Could you check a few things on this drawing? It's one solid part, dimensions in mm from its lowest x, y, z. A direction names the side the tool comes from. Give positions to 0.01 mm unless a question says otherwise; leave off trailing zeros. Loops run counter-clockwise (first coordinate to the right, second up) from the corner with the lowest first, then second, coordinate; pieces in that order, holes last. Notation, with made-up numbers: (-23, 11.5) - (34, 11.5) arc R29 cw to (34, 31.5) - close; hole circle Ø1 at (59.5, 68). An arc over 180 degrees is marked (long way). Use CSV: the item, a comma, the result in double quotes.
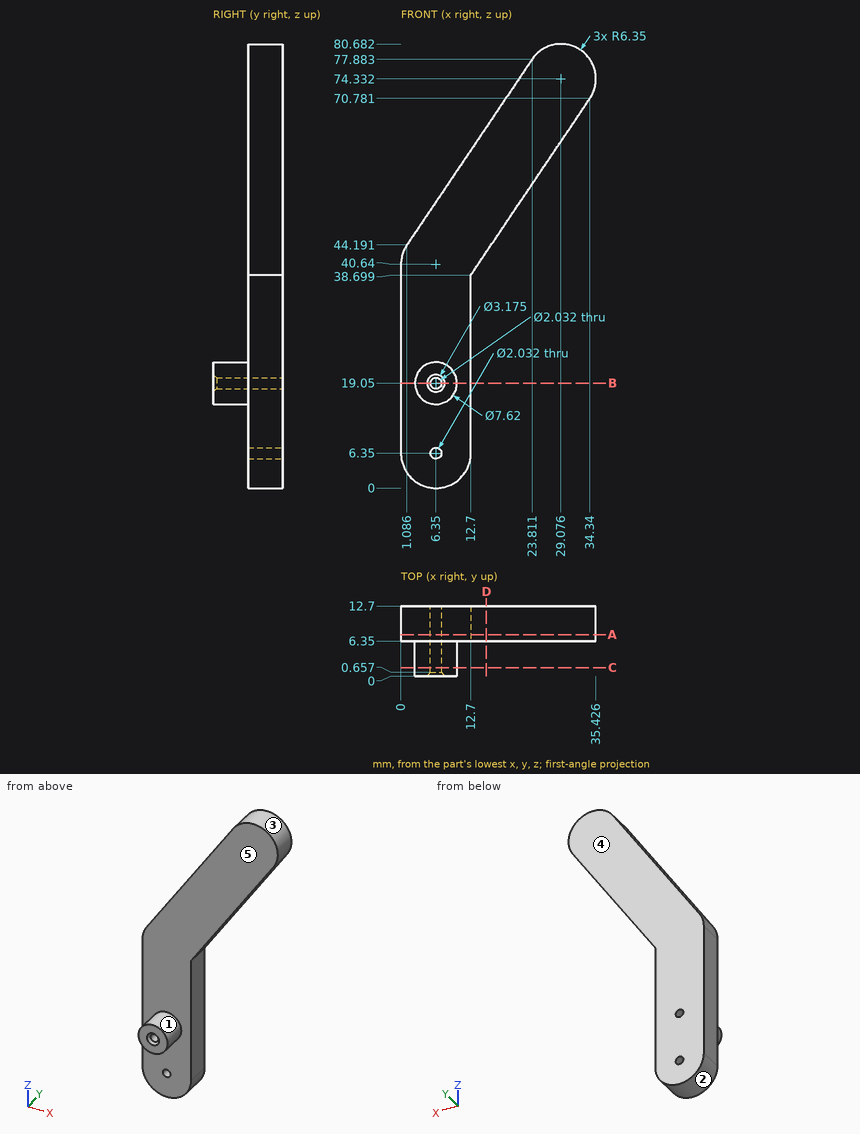
1) Which directions (+Z, -Z, +X, -X, +Y, -Y) give clear straight access to the entire face, cutting with the end or side of a thin tool? Please do the marked faces 1 and 2.
Answer below:
face 1,"-Y"
face 2,"-Z, +Y, -Y"
2) We'd pull the mould along Y, two halves only. Please class the marked faces 3, 4 and 5: +Y half, -Y half, draft (parallel to the pull), parting line (faces both ways), or undercut.
Answer below:
face 3,"draft"
face 4,"+Y half"
face 5,"-Y half"
3) Suppose I cut it at D-D (x = 15.5). Please give me the cut outline in (y, z).
Answer below:
outline,"(6.35, 42.85) - (12.7, 42.85) - (12.7, 65.56) - (6.35, 65.56) - close"
4) Suppose I cut it at A-A (y = 7.5). State how many separate pieces and enclosed holes the cut face has, plus the area to 3 significant figures.
Answer below:
separate pieces,"1"
enclosed holes,"2"
area,"1,070 mm2"
5) Suppose I cut it at B-B (z = 19.05). Please give me the cut outline in (x, y), plus the area to 3 significant figures.
Answer below:
outline,"(0, 6.35) - (2.54, 6.35) - (2.54, 0) - (4.76, 0) - (5.33, 0.66) - (5.33, 12.7) - (0, 12.7) - close; (7.37, 0.66) - (7.94, 0) - (10.16, 0) - (10.16, 6.35) - (12.7, 6.35) - (12.7, 12.7) - (7.37, 12.7) - close"
area,"103 mm2"
6) I need wall thicknesses on line 1 along X through (y, z) = (10, 19.05); line 2 along Y through (x, z) = (25.5, 67); line 3 along Z through (x, y) = (6.35, 9) (1 decimal). Which ranges of each line are inside material? Lowest first, please.
Answer below:
line 1,"x = 0 to 5.33, 7.37 to 12.7"
line 2,"y = 6.35 to 12.7"
line 3,"z = 0 to 5.3, 7.4 to 18, 20.1 to 52"
7) Suppose I cut it at C-C (y = 1.5). Please give me the cut outline in (x, z).
Answer below:
outline,"circle Ø7.62 at (6.35, 19.05); hole circle Ø2.03 at (6.35, 19.05)"
8) I'm going to push flat-ended pins straight in: P1, Ø1, axis at x = 18.5, y = 6.5, coming from the +Z side; P2, Ø3, axis at y = 11, z = 55.5, coming from the -X side; P3, Ø4, axis at y = 7.5, z = 42.5, coming from the +X side; P4, Ø3.5, axis at x = 6.35, z = 6.35, coming from the +Y side. Where does each tip first touch, or does it pass through?
Answer below:
P1,"stops at z = 70.75"
P2,"stops at x = 7.7"
P3,"stops at x = 16.61"
P4,"stops at y = 12.7"
